```python
from build123d import *

# Parameters (mm, degrees)
F0_W     = 137.367442
F0_H     = 108.906533
F1_DEPTH = 76.2
F2_T     = -2.54


with BuildPart() as f1:
    # F0 (on Top) → F1 (new body)
    with BuildSketch(Plane.XY):
        with Locations((-2.032921, -2.178131)):
            Rectangle(F0_W, F0_H)
    extrude(amount=F1_DEPTH)

    # F2
    f2_openings = [f1.faces().sort_by_distance(p)[0] for p in [
        (-2.032921, -2.178131, 76.2),
    ]]
    offset(amount=F2_T, openings=f2_openings)


solid = f1.part
```
Build history of the part. All positions in model axes, mm. A direction names the side the tool comes from. Round coordinates to 2 decimals unless told otherwise and drop trailing zeros. Write each loop counter-clockwise with the first axis right and the second up, starting at its lowest first coordinate (ties: lowest second). Pieces come first, ordered by that corner, then holes.
1) Mould opens along Y. For faces 3 (the flat face through (-68.177, -3, 39)), 4 (the flat face through (66.651, -3, 38)), 5 (the flat face through (-3, -56.631, 38)) say: +Y half, -Y half, draft (parallel to the pull), parting line (faces both ways), or undercut.
2) Band-saw the part on B-B, the plane y = 16. List the corners of the cut face in (x, z), and give its area (3 significant figures).
3) Drill centre lines: probe 1 along Y at (x, z) = (48.5, 45); probe 2 along X at (y, z) = (10, 46); probe 3 along Z at (x, y) = (-13.5, 34). Where is each one in solid material? Low to high.
4) Band-saw the part on C-C, the plane x = -13. List the corners of the cut face in (y, z), and give its area (3 significant figures).
5) Band-saw the part on A-A, the plane z = 25. List the corners of the cut face in (x, y), and give its area (3 significant figures).
6) 3-axis set-ups, long thin cutter, end or side, ignore diameter. For faces 1 (the flat face through (-68.5, -1.9, 76.2)), 2 (the flat face through (-3, 49.735, 39)): which of +Z, -Z, +X, -X, +Y, -Y reach the whole face in a straight line?
7) Pin check, flat tip, straight feed: pin 1 (10 mm diameter, centred on x = -32, y = 15, fed in from +Z). Stop position of the tip, or through.
Ans:
1. face 3: undercut
1. face 4: draft
1. face 5: -Y half
2. outline: (-70.72, 0) - (66.65, 0) - (66.65, 76.2) - (64.11, 76.2) - (64.11, 2.54) - (-68.18, 2.54) - (-68.18, 76.2) - (-70.72, 76.2) - close
2. area: 723 mm2
3. probe 1: y = -56.63 to -54.09, 49.74 to 52.28
3. probe 2: x = -70.72 to -68.18, 64.11 to 66.65
3. probe 3: z = 0 to 2.54
4. outline: (-56.63, 0) - (52.28, 0) - (52.28, 76.2) - (49.74, 76.2) - (49.74, 2.54) - (-54.09, 2.54) - (-54.09, 76.2) - (-56.63, 76.2) - close
4. area: 651 mm2
5. outline: (-70.72, -56.63) - (66.65, -56.63) - (66.65, 52.28) - (-70.72, 52.28) - close; hole (-68.18, -54.09) - (64.11, -54.09) - (64.11, 49.74) - (-68.18, 49.74) - close
5. area: 1,230 mm2
6. face 1: +Z, +X, -X, +Y, -Y
6. face 2: +Z
7. pin 1: stops at z = 2.54
